Check sheet for the modelled part. Datum: model origin and axes. Units: mm. A direction names the side the tool comes from. Round coordinates to 2 decimals unless told otherwise and drop trailing zeros. Write each loop counter-clockwise with the first axis right and the second up, starting at its lowest first coordinate (ties: lowest second). Pieces come first, ordered by that corner, then holes.
Item 1: Material ranges on line 1 (Y direction, x = -5, z = 2.4); line 2 (X direction, y = 14, z = 2.8); line 3 (X direction, y = -20, z = 3.5), recorded low to high.
Item 2: Cross-section at A-A on y = -7. Enter the section's corners in (x, z), plus the area to 3 significant figures.
Item 3: Cross-section at C-C on y = 14.3. Enter the section's corners in (x, z), plus the area to 3 significant figures.
Item 4: Cross-section at B-B on x = -5. Enter the section's corners in (y, z).
Item 5: Tool access check on faces 1 (the flat face through (-1, 45, 2)), 2 (the flat face through (0, 10, 3)). Record the directions out of +Z, -Z, +X, -X, +Y, -Y that give a thin tool (end or side, any length) a straight path to the whole face; none if there is none.
Item 6: Release check for a two-part mould opening along X. For faces 3 (the flat face through (0, -30, 3)), 4 (the flat face through (10, -10, 3)), 5 (the cylindrical face through (-43.289, -43.196, 2.535)), 6 (the flat face through (-1, 11, 5)) record: +X half, -X half, draft (parallel to the pull), parting line (faces both ways), or undercut.
from build123d import *

# Parameters (mm, degrees)
SKETCH_W        = 90
SKETCH_H        = 90
PAD_DEPTH       = 5
SKETCH001_R     = 1.55
POCKET_DEPTH    = 5
FILLET_R        = 6
SKETCH002_W     = 20
SKETCH002_H     = 40
POCKET001_DEPTH = 5
SKETCH003_R     = 2.25
POCKET002_DEPTH = 5


with BuildPart() as part:
    # Sketch → Pad (new body)
    with BuildSketch(Plane.XY):
        Rectangle(SKETCH_W, SKETCH_H)
    extrude(amount=PAD_DEPTH)

    # Sketch001 (on Face6 of Pad) → Pocket (cut)
    with BuildSketch(Plane.XY.offset(5)):
        with Locations((-40, 40)):
            Circle(SKETCH001_R)
        with Locations((40, 40)):
            Circle(SKETCH001_R)
        with Locations((40, -40)):
            Circle(SKETCH001_R)
        with Locations((-40, -40)):
            Circle(SKETCH001_R)
    extrude(amount=-POCKET_DEPTH, mode=Mode.SUBTRACT)

    # Fillet
    fillet_edges = [part.edges().sort_by_distance(p)[0] for p in [
        (-45, -45, 2.5),
        (45, -45, 2.5),
        (45, 45, 2.5),
        (-45, 45, 2.5),
    ]]
    fillet(fillet_edges, radius=FILLET_R)

    # Sketch002 (on Face5 of Fillet) → Pocket001 (cut)
    with BuildSketch(Plane.XY.offset(5)):
        with Locations((0, -10)):
            Rectangle(SKETCH002_W, SKETCH002_H)
    extrude(amount=-POCKET001_DEPTH, mode=Mode.SUBTRACT)

    # Sketch003 (on Face5 of Pocket001) → Pocket002 (cut)
    with BuildSketch(Plane.XY.offset(5)):
        with Locations((-5, 14.3)):
            Circle(SKETCH003_R)
        with Locations((5, 14.3)):
            Circle(SKETCH003_R)
        with Locations((-5, -34.3)):
            Circle(SKETCH003_R)
        with Locations((5, -34.3)):
            Circle(SKETCH003_R)
    extrude(amount=-POCKET002_DEPTH, mode=Mode.SUBTRACT)


solid = part.part
Response values:
1. line 1: y = -45 to -36.55, -32.05 to -30, 10 to 12.05, 16.55 to 45
1. line 2: x = -45 to -7.23, -2.77 to 2.77, 7.23 to 45
1. line 3: x = -45 to -10, 10 to 45
2. outline: (-45, 0) - (-10, 0) - (-10, 5) - (-45, 5) - close; (10, 0) - (45, 0) - (45, 5) - (10, 5) - close
2. area: 350 mm2
3. outline: (-45, 0) - (-7.25, 0) - (-7.25, 5) - (-45, 5) - close; (-2.75, 0) - (2.75, 0) - (2.75, 5) - (-2.75, 5) - close; (7.25, 0) - (45, 0) - (45, 5) - (7.25, 5) - close
3. area: 405 mm2
4. outline: (-45, 0) - (-36.55, 0) - (-36.55, 5) - (-45, 5) - close; (-32.05, 0) - (-30, 0) - (-30, 5) - (-32.05, 5) - close; (10, 0) - (12.05, 0) - (12.05, 5) - (10, 5) - close; (16.55, 0) - (45, 0) - (45, 5) - (16.55, 5) - close
5. face 1: +Z, -Z, +X, -X, +Y
5. face 2: +Z, -Z
6. face 3: undercut
6. face 4: undercut
6. face 5: -X half
6. face 6: draft
